CAD build for the part. Positions are in the model's coordinates, mm. Face numbers are marked on the shaded views. A direction names the side the tool comes from. Round coordinates to 2 decimals unless told otherwise and drop trailing zeros. Loops run counter-clockwise (first coordinate to the right, second up) from the corner with the lowest first, then second, coordinate; pieces in that order, holes last. Notation, with made-up numbers: (-29, 54) -> (-5, 54) arc R29 cw to (-5, 87) -> close; hole circle Ø2 at (-9, 60.5). An arc over 180 degrees is marked (long way). Answer as CSV lines item,"result".
```python
from build123d import *

# Parameters (mm, degrees)
BOSS_EXTRUDE1_DEPTH = 60
SKETCH2_R           = 2.75
CUT_EXTRUDE1_DEPTH  = 6
FILLET1_R           = 3


with BuildPart() as part:
    # Sketch1 → Boss-Extrude1 (new body)
    with BuildSketch(Plane.XY):
        with BuildLine():
            Line((-11.15, 0), (-11.15, -11.15))
            Line((-11.15, -11.15), (-30, -11.15))
            Line((-30, -11.15), (-30, -5.15))
            Line((-30, -5.15), (-17.15, -5.15))
            Line((-17.15, -5.15), (-17.15, 0))
            ThreePointArc((-17.15, 0), (0, 17.15), (17.15, 0))
            Line((17.15, 0), (17.15, -5.15))
            Line((17.15, -5.15), (30, -5.15))
            Line((30, -5.15), (30, -11.15))
            Line((30, -11.15), (11.15, -11.15))
            Line((11.15, -11.15), (11.15, 0))
            ThreePointArc((11.15, 0), (0, 11.15), (-11.15, 0))
        make_face()
    extrude(amount=BOSS_EXTRUDE1_DEPTH)

    # Sketch2 → Cut-Extrude1 (cut)
    with BuildSketch(Plane(origin=(0, -5.15, 0), x_dir=(1, 0, 0), z_dir=(0, 1, 0))):
        with Locations(Location((-25, -5, 0), (0, 0, 270))):
            Circle(SKETCH2_R)
        with Locations(Location((-25, -55, 0), (0, 0, 90))):
            Circle(SKETCH2_R)
        with Locations(Location((25, -55, 0), (0, 0, 270))):
            Circle(SKETCH2_R)
        with Locations(Location((25, -5, 0), (0, 0, 90))):
            Circle(SKETCH2_R)
    extrude(amount=-CUT_EXTRUDE1_DEPTH, mode=Mode.SUBTRACT)

    # Fillet1
    fillet1_edges = [part.edges().sort_by_distance(p)[0] for p in [
        (-30, -8.15, 0),
        (30, -8.15, 0),
        (30, -8.15, 60),
        (-30, -8.15, 60),
    ]]
    fillet(fillet1_edges, radius=FILLET1_R)


solid = part.part
```
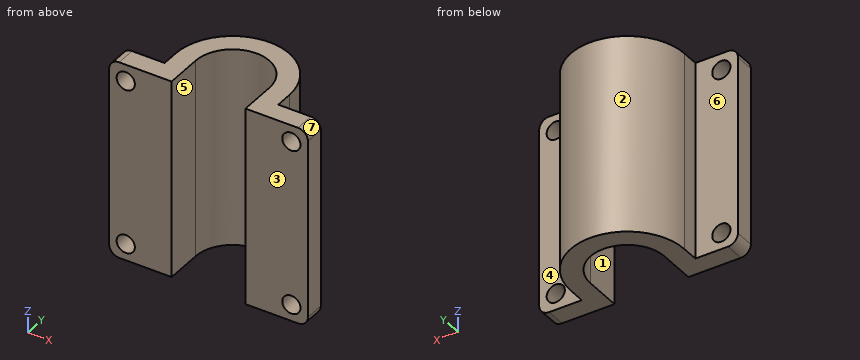
Q1. Drop flat-ended pins along their axis: pin 1 Ø1 at (y, z) = (-4, 44) entering from -X; pin 2 Ø9 at (x, z) = (25, 5) entering from +Y; pin 3 Ø3 at (x, z) = (5.5, 30) entering from -Y. Give the stop position or say it passes through.
Results:
pin 1,"x = -17.15"
pin 2,"y = -5.15"
pin 3,"y = 8.68"
Q2. Tool access for the marked faces 4, 5, 6 and 7: list every direction of +Z, -Z, +X, -X, +Y, -Y with a clear straight run to the whole face (end or side of a thin tool).
Results:
face 4,"+Z, -Z, +X, +Y"
face 5,"+Z, -Z, -Y"
face 6,"+Z, -Z, -X, +Y"
face 7,"+Z, +X, +Y, -Y"
Q3. Slice it at A-A, the plane y = -9.25. Give the cut face in (x, z), and give its area (3 significant figures).
Results:
outline,"(-30, 3) arc R3 ccw to (-27, 0) -> (-11.15, 0) -> (-11.15, 60) -> (-27, 60) arc R3 ccw to (-30, 57) -> close; (11.15, 0) -> (27, 0) arc R3 ccw to (30, 3) -> (30, 57) arc R3 ccw to (27, 60) -> (11.15, 60) -> close; hole circle Ø5.5 at (-25, 5); hole circle Ø5.5 at (-25, 55); hole circle Ø5.5 at (25, 5); hole circle Ø5.5 at (25, 55)"
area,"2,160 mm2"
Q4. Slice it at D-D, the plane z = 13. Give the cut face in (x, y), and give its area (3 significant figures).
Results:
outline,"(-30, -11.15) -> (-11.15, -11.15) -> (-11.15, 0) arc R11.15 cw to (11.15, 0) -> (11.15, -11.15) -> (30, -11.15) -> (30, -5.15) -> (17.15, -5.15) -> (17.15, 0) arc R17.15 ccw to (-17.15, 0) -> (-17.15, -5.15) -> (-30, -5.15) -> close"
area,"555 mm2"
Q5. Two-plate mould, pull along X, no slides. Class the marked faces 1, 2 and 3: pulls with the +X half, pulls with the -X half, needs draft (parallel to the pull), parting line crosses it, or undercut.
Results:
face 1,"undercut"
face 2,"parting line crosses it"
face 3,"needs draft"
Q6. Probe L1, parallel to X at y = -7.55, z = 55; L2, parallel to Z at x = 27, y = -7.75; L3, parallel to X at y = -2.5, z = 25.5. List the from-to ranges inside material, lowest first. Write a range as [from, to].
Results:
L1,"[-30, -27.75], [-22.25, -11.15], [11.15, 22.25], [27.75, 30]"
L2,"[0, 3.11], [6.89, 53.11], [56.89, 60]"
L3,"[-17.15, -11.15], [11.15, 17.15]"
Q7. Slice it at C-C, the plane z = 5. Give the cut face in (x, y), and give its area (3 significant figures).
Results:
outline,"(-30, -11.15) -> (-27.75, -11.15) -> (-27.75, -5.15) -> (-30, -5.15) -> close; (-22.25, -11.15) -> (-11.15, -11.15) -> (-11.15, 0) arc R11.15 cw to (11.15, 0) -> (11.15, -11.15) -> (22.25, -11.15) -> (22.25, -5.15) -> (17.15, -5.15) -> (17.15, 0) arc R17.15 ccw to (-17.15, 0) -> (-17.15, -5.15) -> (-22.25, -5.15) -> close; (27.75, -11.15) -> (30, -11.15) -> (30, -5.15) -> (27.75, -5.15) -> close"
area,"489 mm2"
Q8. Slice it at B-B, the plane x = 25. Give the cut face in (y, z), and give its area (3 significant figures).
Results:
outline,"(-11.15, 0) -> (-5.15, 0) -> (-5.15, 2.25) -> (-11.15, 2.25) -> close; (-11.15, 7.75) -> (-5.15, 7.75) -> (-5.15, 52.25) -> (-11.15, 52.25) -> close; (-11.15, 57.75) -> (-5.15, 57.75) -> (-5.15, 60) -> (-11.15, 60) -> close"
area,"294 mm2"
